```python
from build123d import *

# Parameters (mm, degrees)
SKETCH1_R           = 10
BOSS_EXTRUDE1_DEPTH = 2.5
SKETCH2_R           = 15
SKETCH2_R_2         = 10
BOSS_EXTRUDE2_DEPTH = 15
SKETCH3_R           = 5
CUT_EXTRUDE1_DEPTH  = 74.739406019
BOSS_EXTRUDE3_START = 9.5
SKETCH4_R           = 10
SKETCH4_R_2         = 6
BOSS_EXTRUDE3_DEPTH = 3


with BuildPart() as part:
    # Sketch1 → Boss-Extrude1 (new, symmetric)
    with BuildSketch(Plane(origin=(0, 0, 0), x_dir=(1, 0, 0), z_dir=(0, 1, 0))):
        with BuildLine():
            Line((-12.5, 12.5), (-62.5, 7.5))
            ThreePointArc((-62.5, 7.5), (-70, 0), (-62.5, -7.5))
            Line((-62.5, -7.5), (-12.5, -12.5))
            ThreePointArc((-12.5, -12.5), (17.67766953, 0), (-12.5, 12.5))
        make_face()
        with Locations(Location((0, 0, 0), (0, 0, 270))):
            Circle(SKETCH1_R, mode=Mode.SUBTRACT)
    extrude(amount=BOSS_EXTRUDE1_DEPTH, both=True)

    # Sketch2 → Boss-Extrude2 (add)
    with BuildSketch(Plane(origin=(0, 2.5, 0), x_dir=(1, 0, 0), z_dir=(0, 1, 0))):
        with Locations(Location((0, 0, 0), (0, 0, 270))):
            Circle(SKETCH2_R)
        with Locations(Location((0, 0, 0), (0, 0, 270))):
            Circle(SKETCH2_R_2, mode=Mode.SUBTRACT)
    extrude(amount=BOSS_EXTRUDE2_DEPTH)

    # Sketch3 → Cut-Extrude1 (cut, through all)
    with BuildSketch(Plane(origin=(0, 2.5, 0), x_dir=(1, 0, 0), z_dir=(0, 1, 0))):
        with Locations(Location((-54.417236445, 0, 0), (0, 0, 270))):
            Circle(SKETCH3_R)
    extrude(amount=-CUT_EXTRUDE1_DEPTH, mode=Mode.SUBTRACT)

    # Sketch4 → Boss-Extrude3 (add)
    with BuildSketch(Plane(origin=(0, 0, 0), x_dir=(1, 0, 0), z_dir=(0, 1, 0)).offset(BOSS_EXTRUDE3_START)):
        with Locations(Location((0, 0, 0), (0, 0, 270))):
            Circle(SKETCH4_R)
        with Locations(Location((0, 0, 0), (0, 0, 270))):
            Circle(SKETCH4_R_2, mode=Mode.SUBTRACT)
    extrude(amount=BOSS_EXTRUDE3_DEPTH)


solid = part.part
```
Read the model definition and answer for the solid it produces. Units are mm, in the model's axes. A direction names the side the tool comes from. Round coordinates to 2 decimals unless told otherwise and drop trailing zeros. Write each loop counter-clockwise with the first axis right and the second up, starting at its lowest first coordinate (ties: lowest second). Pieces come first, ordered by that corner, then holes. Notation, with made-up numbers: M 25,13.5 L 42,13.5 A19 ccw 42,42.5 Z; hole C 61.5,67.5 d3. An arc over 180 degrees is marked long. One line per item, written item: value.
Q1. Find section C-C on y = 7.5. Write down the section's boundary in (x, z), plus the area to 3 significant figures.
Data:
outline: C 0,0 d30; hole C 0,0 d20
area: 393 mm2
Q2. Find section A-A on x = 0. Write down the section's boundary in (y, z), plus the area to 3 significant figures.
Data:
outline: M -2.5,-17.68 L 2.5,-17.68 L 2.5,-15 L 17.5,-15 L 17.5,-10 L 12.5,-10 L 12.5,-6 L 9.5,-6 L 9.5,-10 L -2.5,-10 Z; M -2.5,10 L 9.5,10 L 9.5,6 L 12.5,6 L 12.5,10 L 17.5,10 L 17.5,15 L 2.5,15 L 2.5,17.68 L -2.5,17.68 Z
area: 251 mm2
Q3. Find section D-D on z = -4. Write down the section's boundary in (x, y).
Data:
outline: M -68.84,-2.5 L -57.42,-2.5 L -57.42,2.5 L -68.84,2.5 Z; M -51.42,-2.5 L -9.17,-2.5 L -9.17,9.5 L -4.47,9.5 L -4.47,12.5 L -9.17,12.5 L -9.17,17.5 L -14.46,17.5 L -14.46,2.5 L -51.42,2.5 Z; M 4.47,9.5 L 9.17,9.5 L 9.17,-2.5 L 17.22,-2.5 L 17.22,2.5 L 14.46,2.5 L 14.46,17.5 L 9.17,17.5 L 9.17,12.5 L 4.47,12.5 Z
Q4. For a pull along X with two mould halves and no side action, classify faces 1 (the flat face through (-27, 2.5, 0)), 2 (the flat face through (-37.85, 0.035, 9.965)), 3 (the cylindrical face through (-9.76, 3.42, -2.17)), 4 (the cylindrical face through (17.67, 0.04, 0.58)) as +X half, -X half, draft (parallel to the pull), parting line (faces both ways), or undercut.
Data:
face 1: draft
face 2: -X half
face 3: undercut
face 4: parting line
Q5. Which of the six approach directions +Z, -Z, +X, -X, +Y, -Y give full straight-line access (tool end or side, diameter ignored) to faces 5 (the flat face through (-17, -2.5, 0)), 6 (the cylindrical face through (0.66, 9.895, -14.985)), 7 (the flat face through (-7, 9.5, 0))?
Data:
face 5: +Z, -Z, +X, -X, -Y
face 6: +Y
face 7: -Y
Q6. Find section B-B on z = 0. Write down the section's boundary in (x, y).
Data:
outline: M -70,-2.5 L -59.42,-2.5 L -59.42,2.5 L -70,2.5 Z; M -49.42,-2.5 L -10,-2.5 L -10,9.5 L -6,9.5 L -6,12.5 L -10,12.5 L -10,17.5 L -15,17.5 L -15,2.5 L -49.42,2.5 Z; M 6,9.5 L 10,9.5 L 10,-2.5 L 17.68,-2.5 L 17.68,2.5 L 15,2.5 L 15,17.5 L 10,17.5 L 10,12.5 L 6,12.5 Z
Q7. Flat-ended cylindrical pins translate along their axes: pin 1 Ø3 at (y, z) = (10.5, 13) entering from +X; pin 2 Ø11.5 at (x, z) = (-54.42, 0) entering from +Y; pin 3 Ø5 at (y, z) = (4, 13.5) entering from +X. Find the tip coordinate at first contact, or state that the pin passes through.
Data:
pin 1: x = 9.63
pin 2: y = 2.5
pin 3: x = 13.43
Q8. Straight lines are drawn through the part: line 1 (X direction, y = 1.45, z = 0); line 2 (X direction, y = 14.55, z = 0); line 3 (X direction, y = 10.9, z = 0). For each, find the intervals that lie inside material, in ascending order. Write a range as [from, to].
Data:
line 1: [-70, -59.42], [-49.42, -10], [10, 17.68]
line 2: [-15, -10], [10, 15]
line 3: [-15, -6], [6, 15]
